Here's how the part is built. I have some questions about the finished solid (model axes, mm). Face numbers are marked on the shaded views. A direction names the side the tool comes from. Coordinates: 2 decimals unless noted, no trailing zeros. Order: outer loops, then holes, each group sorted by start corner. A loop starts at its lowest first (then second) coordinate and runs counter-clockwise, first axis right, second up.
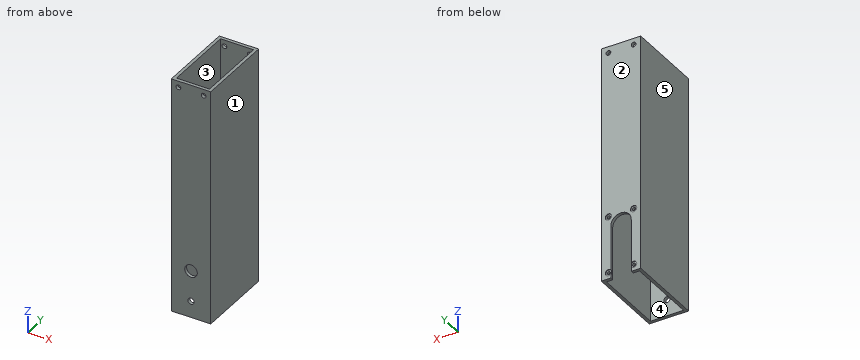
Autodesk Inventor part; units mm, degrees
ref_plane "YZ Plane" through (0, 0, 0) normal (1, 0, 0) x (0, 1, 0)
ref_plane "XZ Plane" through (0, 0, 0) normal (0, 1, 0) x (-1, 0, 0)
ref_plane "XY Plane" through (0, 0, 0) normal (0, 0, 1) x (1, 0, 0)
sketch "スケッチ1" plane through (0, 0, 0) normal (0, 0, 1) x (1, 0, 0)
  line L0 (-12.5, 25) -> (12.5, 25)
  line L1 (12.5, 25) -> (12.5, -25)
  line L2 (12.5, -25) -> (-12.5, -25)
  line L3 (-12.5, -25) -> (-12.5, 25)
  line L4 (-10.5, 23) -> (10.5, 23)
  line L5 (10.5, 23) -> (10.5, -23)
  line L6 (10.5, -23) -> (-10.5, -23)
  line L7 (-10.5, -23) -> (-10.5, 23)
  point P0 (0, 0)
  dimension "d0" = 25
  dimension "d1" = 50
  dimension "d2" = 46
  dimension "d3" = 21
  dimension "d4" = 25
  dimension "d5" = 23
  dimension "d6" = 10.5
  dimension "d7" = 12.5
extrude "押し出し1" add sketch "スケッチ1" along normal blind 150
sketch "スケッチ2" plane through (-12.5, 25, 0) normal (0, 1, 0) x (1, 0, 0)
  line L0 (0, 0) -> (25, 0)
  line L1 (0, 0) -> (0, -150)
  arc A0 (6, -33.5) -> (19, -33.5) centre (12.5, -33.5) ccw
  line L2 (6, -33.5) -> (6, 0)
  line L3 (19, -33.5) -> (19, 0)
  point P0 (12.5, 0)
  dimension "d10" = 13
  dimension "d11" = 33.5
  dimension "d12" = 12.5
extrude "押し出し2" cut sketch "スケッチ2" against normal blind 2
sketch "スケッチ3" plane through (-12.5, 25, 150) normal (0, 1, 0) x (1, 0, 0)
  arc A0 (6, 116.5) -> (19, 116.5) centre (12.5, 116.5) ccw
  circle A1 centre (4.5, 110) radius 1
  circle A2 centre (4.5, 146) radius 1
  circle A3 centre (20.5, 146) radius 1
  circle A4 centre (20.5, 110) radius 1
  point P0 (12.5, 150)
  dimension "d15" = 6.5
  dimension "d16" = 6.5
  dimension "d17" = 2
  dimension "d18" = 8
  dimension "d19" = 8
  dimension "d20" = 8
  dimension "d21" = 8
  dimension "d22" = 29.5
  dimension "d23" = 29.5
hole "穴1" at (-8, 25, 4) at (8, 25, 4) at (8, 25, 40) at (-8, 25, 40) direction (0, -1, 0) diameter 2 depth 2 tip angle 118 counterbore diameter 4 counterbore depth 0.5
sketch "スケッチ4" plane through (-12.5, -25, 0) normal (0, -1, 0) x (1, 0, 0)
  line L0 (25, 0) -> (0, 0)
  line L1 (25, 0) -> (25, 150)
  circle A0 centre (12.5, 10.5) radius 2
  point P0 (12.5, 0)
  dimension "d31" = 4
  dimension "d32" = 12.5
  dimension "d33" = 10.5
hole "穴2" at (0, -25, 10.5) direction (0, 1, 0) diameter 4 end through all
sketch "スケッチ5" plane through (-12.5, 25, 150) normal (0, 1, 0) x (1, 0, 0)
  line L0 (0, 0) -> (25, 0)
  arc A0 (6, 116.5) -> (19, 116.5) centre (12.5, 116.5) ccw
  circle A1 centre (20.5, 4) radius 1.5
  circle A2 centre (4.5, 4) radius 1.5
  point P0 (12.5, 150)
  dimension "d43" = 4
  dimension "d44" = 4
  dimension "d46" = 8
  dimension "d47" = 8
  dimension "d57" = 3
hole "穴4" at (-8, 25, 146) at (8, 25, 146) direction (0, -1, 0) diameter 3 end through all
thread "ねじ1"
thread "ねじ2"
thread "ねじ3"
thread "ねじ4"
sketch "スケッチ7" plane through (-12.5, -25, 0) normal (0, -1, 0) x (1, 0, 0)
  line L0 (25, 0) -> (25, 150)
  circle A0 centre (12.5, 30) radius 4
  line L1 (25, 0) -> (0, 0)
  point P0 (12.5, 0)
  dimension "d79" = 8
  dimension "d80" = 12.5
  dimension "d88" = 30
hole "穴5" at (0, -25, 30) direction (0, 1, 0) diameter 8 end through all
properties part number "07" material "アルミニウム 6061"
Q1. I need wall thicknesses on L1, parallel to Z at x = -8, y = 24.8; L2, parallel to Z at x = -8, y = 23.45; L3, parallel to Y at x = -8.25, z = 17.5. Which ranges of each line are inside material? Lowest first, please.
Q2. If we section it at D-D on z = 62: Write out the boundary of the cut face in (x, y), then the cut area to 3 significant figures.
Q3. Will these pins go through, and if not, where does the flat tip stop? pin 1 (4.5 mm diameter, centred on x = -7.5, z = 39.5, fed in from +Y); pin 2 (2.5 mm diameter, centred on x = -8, z = 4, fed in from +Y); pin 3 (2.5 mm diameter, centred on x = 8, z = 146, fed in from +Y); pin 4 (1 mm diameter, centred on x = 8, z = 4, fed in from +Y).
Q4. If we section it at A-A on z = 10.5: Write out the boundary of the cut face in (x, y), then the cut area to 3 significant figures.
Q5. For the marked faces 4 and 5, which set-ups out of +Z, -Z, +X, -X, +Y, -Y let a thin tool reach every point of the face, with its end or its side?
Q6. If we section it at C-C on x = 0: Write out the boundary of the cut face in (y, z), then the cut area to 3 significant figures.
Q7. If we section it at B-B on y = 21.5: Write out the boundary of the cut face in (x, z).
Q8. We'd pull the mould along X, two halves only. Please class the marked faces 1, 2 and 3: pulls with the +X half, pulls with the -X half, needs draft (parallel to the pull), parting line crosses it, or undercut.
Reply:
1. L1: z = 0 to 2, 6 to 38, 42 to 144.5, 147.5 to 150
1. L2: z = 0 to 3, 5 to 39, 41 to 144.5, 147.5 to 150
1. L3: y = -25 to -23, 23 to 25
2. outline: (-12.5, -25) - (12.5, -25) - (12.5, 25) - (-12.5, 25) - close; hole (-10.5, -23) - (10.5, -23) - (10.5, 23) - (-10.5, 23) - close
2. area: 284 mm2
3. pin 1: stops at y = 25
3. pin 2: stops at y = 24.5
3. pin 3: passes through
3. pin 4: stops at y = -23
4. outline: (-12.5, -25) - (-2, -25) - (-2, -23) - (-10.5, -23) - (-10.5, 23) - (-6.5, 23) - (-6.5, 25) - (-12.5, 25) - close; (2, -25) - (12.5, -25) - (12.5, 25) - (6.5, 25) - (6.5, 23) - (10.5, 23) - (10.5, -23) - (2, -23) - close
4. area: 250 mm2
5. face 4: +Z, -Z
5. face 5: +Z, -Z, -X, +Y, -Y
6. outline: (-25, 0) - (-23, 0) - (-23, 8.5) - (-25, 8.5) - close; (-25, 12.5) - (-23, 12.5) - (-23, 26) - (-25, 26) - close; (-25, 34) - (-23, 34) - (-23, 150) - (-25, 150) - close; (23, 40) - (25, 40) - (25, 150) - (23, 150) - close
6. area: 496 mm2
7. outline: (-12.5, 0) - (-10.5, 0) - (-10.5, 150) - (-12.5, 150) - close; (10.5, 0) - (12.5, 0) - (12.5, 150) - (10.5, 150) - close
8. face 1: pulls with the +X half
8. face 2: needs draft
8. face 3: undercut
